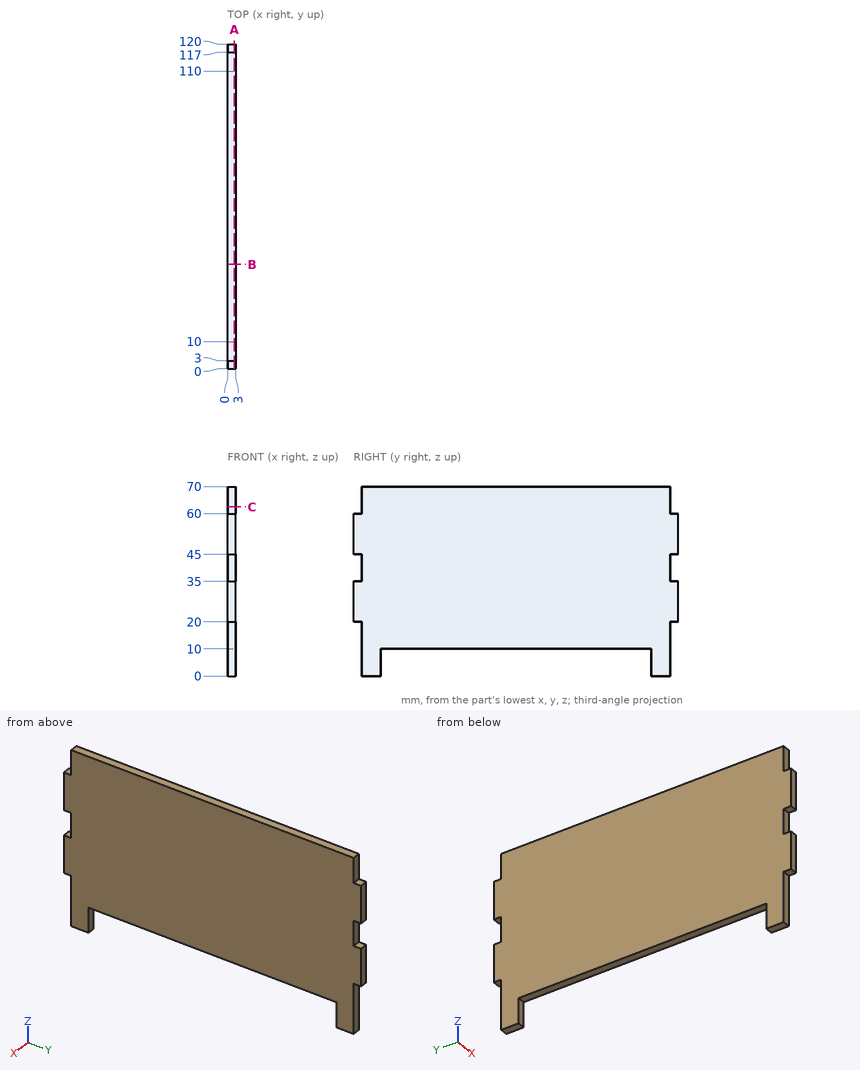
Verification items for this drawing (mm, ordinates from the low corner). Coordinates: 2 decimals unless noted, no trailing zeros. Order: outer loops, then holes, each group sorted by start corner. A loop starts at its lowest first (then second) coordinate and runs counter-clockwise, first axis right, second up. Notation, with made-up numbers: (-21.5, 56) -> (-17.5, 56) arc R32 cw to (-17.5, 88) -> close; hole circle Ø7 at (5, 83.5). An arc over 180 degrees is marked (long way). Put each result on its own line as item: value. Start each with the question number.
1. Go/stop test with flat-tipped pins: pin 1 Ø0.9 at (x, y) = (1.5, 119) entering from -Z; pin 2 Ø1.5 at (x, y) = (2, 119) entering from +Z; pin 3 Ø0.9 at (x, z) = (1, 40) entering from +Y. Record where each tip stops, or that it passes through.
2. Cross-section at A-A, the plane x = 2.5. Record the boundary of the cut face in (y, z).
3. Material ranges on L1, parallel to Y at x = 2.15, z = 38.5; L2, parallel to Z at x = 2.75, y = 87, recorded low to high. Write a range as [from, to].
4. Cross-section at C-C, the plane z = 62.5. Record the boundary of the cut face in (x, y), then the cut area to 3 significant figures.
5. Cross-section at B-B, the plane y = 38.5. Record the boundary of the cut face in (x, z).
Computed:
1. pin 1: z = 20
1. pin 2: z = 60
1. pin 3: y = 117
2. outline: (0, 20) -> (3, 20) -> (3, 0) -> (10, 0) -> (10, 10) -> (110, 10) -> (110, 0) -> (117, 0) -> (117, 20) -> (120, 20) -> (120, 35) -> (117, 35) -> (117, 45) -> (120, 45) -> (120, 60) -> (117, 60) -> (117, 70) -> (3, 70) -> (3, 60) -> (0, 60) -> (0, 45) -> (3, 45) -> (3, 35) -> (0, 35) -> close
3. L1: [3, 117]
3. L2: [10, 70]
4. outline: (0, 3) -> (3, 3) -> (3, 117) -> (0, 117) -> close
4. area: 342 mm2
5. outline: (0, 10) -> (3, 10) -> (3, 70) -> (0, 70) -> close
